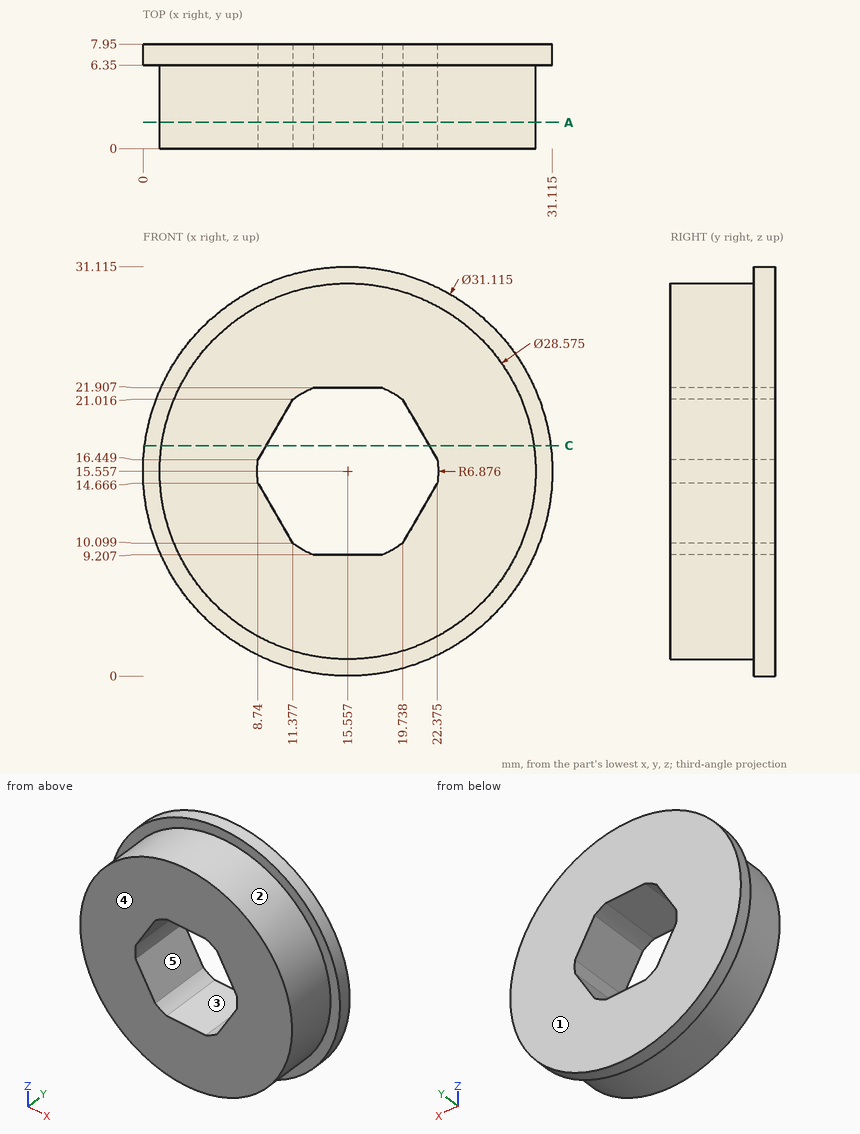
Print and shaded views of the part. All mm, measured from the part's lowest x, y and z. A direction names the side the tool comes from. Give positions to 0.01 mm unless a question says otherwise; leave off trailing zeros. Write each loop counter-clockwise with the first axis right and the second up, starting at its lowest first coordinate (ties: lowest second). Pieces come first, ordered by that corner, then holes. Notation, with made-up numbers: (-12.75, -12) - (22.25, -12) arc R20 ccw to (22.25, 12) - close; hole circle Ø2 at (-21, 12.25). An arc over 180 degrees is marked (long way). One line per question, with ' | ' between items. Start each with the question number.
(1) 3-axis set-ups, long thin cutter, end or side, ignore diameter. For the marked faces 4 and 5: which of +Z, -Z, +X, -X, +Y, -Y reach the whole face in a straight line?
(2) Pin check, flat tips, straight feed: P1, Ø1.5, axis at x = 10, y = 7, coming from the -Z side; P2, Ø1.6, axis at x = 15.5, y = 2, coming from the +Z side (1 decimal); P3, Ø1, axis at x = 5.5, z = 4, coming from the -Y side. Stop position of each tip, or through.
(3) Slice it at C-C on z = 17.5. Write the cut outline in (x, y).
(4) Wall check: line 1 along X through (y, z) = (7, 14.5) (1 decimal); line 2 along Y through (x, z) = (24, 28.5); line 3 along Z through (x, y) = (17, 4.5). Give the ranges that are in metal, low to high. Write a range as from..to.
(5) Slice it at A-A on y = 2. Write the cut outline in (x, z) (1 decimal).
(6) Two-plate mould, pull along Z, no slides. Class the marked faces 1, 2 and 3: +Z half, -Z half, draft (parallel to the pull), parting line (faces both ways), or undercut.
Results below:
1) face 4: +Z, -Z, +X, -X, -Y | face 5: +Y, -Y
2) P1: z = 0.76 | P2: z = 29.8 | P3: y = 6.35
3) outline: (0.12, 6.35) - (1.4, 6.35) - (1.4, 0) - (9.35, 0) - (9.35, 7.95) - (0.12, 7.95) - close; (21.77, 0) - (29.71, 0) - (29.71, 6.35) - (30.99, 6.35) - (30.99, 7.95) - (21.77, 7.95) - close
4) line 1: 0..8.8, 22.3..31.1 | line 2: 6.35..7.95 | line 3: 1.34..9.21, 21.91..29.77
5) outline: circle Ø28.6 at (15.6, 15.6); hole (8.7, 14.7) - (11.4, 10.1) arc R6.9 ccw to (12.9, 9.2) - (18.2, 9.2) arc R6.9 ccw to (19.7, 10.1) - (22.4, 14.7) arc R6.9 ccw to (22.4, 16.4) - (19.7, 21) arc R6.9 ccw to (18.2, 21.9) - (12.9, 21.9) arc R6.9 ccw to (11.4, 21) - (8.7, 16.4) arc R6.9 ccw to start
6) face 1: draft | face 2: parting line | face 3: undercut
